Geometry: final body of the model. Coordinates: model frame, mm. Face numbers are marked on the shaded views. A direction names the side the tool comes from. Give positions to 0.01 mm unless a question says otherwise; leave off trailing zeros. Order: outer loops, then holes, each group sorted by start corner. A loop starts at its lowest first (then second) coordinate and runs counter-clockwise, first axis right, second up. Notation, with made-up numbers: (11, 72.5) -> (21, 72.5) arc R18 ccw to (21, 101.5) -> close; hole circle Ø8 at (4, 12). An arc over 180 degrees is marked (long way). Write item = value, one per line.
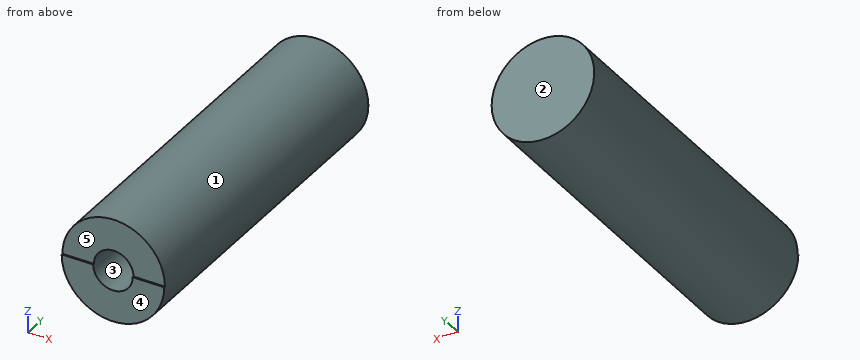
```python
from build123d import *

# Parameters (mm, degrees)
F0_R     = 82.2325
F1_DEPTH = 545.338
F2_R     = 31.75
F3_DEPTH = 385.318
F4_R     = 0.889
F6_DEPTH = 2


with BuildPart() as f1:
    # F0 (on Front) → F1 (new body)
    with BuildSketch(Plane.XZ):
        Circle(F0_R)
    extrude(amount=F1_DEPTH)

    # F2 (on face) → F3 (cut)
    with BuildSketch(Plane.XZ.offset(545.338)):
        Circle(F2_R)
    extrude(amount=-F3_DEPTH, mode=Mode.SUBTRACT)

    # F4
    f4_edges = [f1.edges().sort_by_distance(p)[0] for p in [
        (-31.75, -160.02, 0),
    ]]
    fillet(f4_edges, radius=F4_R)

    # F5 (on face) → F6 (cut)
    with BuildSketch(Plane.XZ.offset(545.338)):
        Polygon((-94.683126, 74.995518), (-90.933107, 0), (99.84915, 0), (85.317813, 66.08922), (21.098729, 103.589416), (-59.526693, 95.151864), align=None)
    extrude(amount=-F6_DEPTH, mode=Mode.SUBTRACT)


solid = f1.part
```
1) Section query C-C (x = -71). Output: boundary loops of the cut face in (y, z).
Check sheet entries:
outline = (-545.34, -41.49) -> (0, -41.49) -> (0, 41.49) -> (-543.34, 41.49) -> (-543.34, 0) -> (-545.34, 0) -> close
2) First-contact query: P1, Ø3, axis at y = -456.5, z = -62, coming from the -X side (3 decimals); P2, Ø8, axis at x = 24, y = -461.5, coming from the -Z side; P3, Ø12, axis at x = 11.5, y = -403, coming from the +Z side. Flat tips, straight axial feed; report the tip coordinate or a pass-through.
Check sheet entries:
P1 = -55.695
P2 = -79.76
P3 = 82.05
3) Mould query, pull axis X, two halves, no side actions, for the marked faces 1, 2 and 3. Classes: +X half, -X half, draft (parallel to the pull), parting line (faces both ways), or undercut.
Check sheet entries:
face_1 = parting line
face_2 = draft
face_3 = undercut
4) Line query: line 1 (X direction, y = -271, z = 0); line 2 (Y direction, x = -61.5, z = 20). Output: solid intervals per line, ascending. Write a range as from..to.
Check sheet entries:
line_1 = -82.23..-31.75, 31.75..82.23
line_2 = -543.34..0
5) Reachability of the marked faces 4 and 5 from +Z, -Z, +X, -X, +Y, -Y: full face, straight path, thin tool, end or side. Return the list, or none.
Check sheet entries:
face_4 = +Z, -Z, +X, -X, -Y
face_5 = +Z, +X, -X, -Y
6) Section query D-D (z = -38). Output: boundary loops of the cut face in (x, y), plus the area to 3 significant figures.
Check sheet entries:
outline = (-72.93, -545.34) -> (72.93, -545.34) -> (72.93, 0) -> (-72.93, 0) -> close
area = 79,500 mm²
7) Section query B-B (x = 0). Output: boundary loops of the cut face in (y, z).
Check sheet entries:
outline = (-545.34, -82.23) -> (0, -82.23) -> (0, 82.23) -> (-543.34, 82.23) -> (-543.34, 31.75) -> (-160.91, 31.75) arc R0.89 cw to (-160.02, 30.86) -> (-160.02, -30.86) arc R0.89 cw to (-160.91, -31.75) -> (-545.34, -31.75) -> close
